from build123d import *

# Parameters (mm, degrees)
F0_W     = 1828.8
F0_H     = 558.8
F1_DEPTH = 19.05
F2_W     = 38.1
F2_H     = 88.9
F3_DEPTH = 1828.8
F4_W     = 38.1
F4_H     = 88.9
F5_DEPTH = 482.6
F6_W     = 88.9
F6_H     = 38.1
F7_DEPTH = 863.6


with BuildPart() as f1:
    # F0 (on Top) → F1 (new body)
    with BuildSketch(Plane.XY):
        with Locations((914.4, -279.4)):
            Rectangle(F0_W, F0_H)
    extrude(amount=F1_DEPTH)

    # F2 (on face) → F3 (join, through all)
    with BuildSketch(Plane.YZ.offset(1828.8)):
        with Locations((-539.75, -44.45)):
            Rectangle(F2_W, F2_H)
        with Locations((-19.05, -44.45)):
            Rectangle(F2_W, F2_H)
    extrude(amount=-F3_DEPTH)

    # F4 (on face) → F5 (join, through all)
    with BuildSketch(Plane.XZ.offset(38.1)):
        with Locations((19.05, -44.45)):
            Rectangle(F4_W, F4_H)
        with Locations((1809.75, -44.45)):
            Rectangle(F4_W, F4_H)
    extrude(amount=F5_DEPTH)

    # F6 (on face) → F7 (join)
    with BuildSketch(Plane(origin=(0, 0, 0), x_dir=(1, 0, 0), z_dir=(0, 0, -1))):
        with Locations((1746.25, 501.65)):
            Rectangle(F6_W, F6_H)
        with Locations((1746.25, 57.15)):
            Rectangle(F6_W, F6_H)
        with Locations((82.55, 57.15)):
            Rectangle(F6_W, F6_H)
        with Locations((82.55, 501.65)):
            Rectangle(F6_W, F6_H)
    extrude(amount=F7_DEPTH)


solid = f1.part
Verification items for the finished model (mm, model axes). A direction names the side the tool comes from. Give positions to 0.01 mm unless a question says otherwise; leave off trailing zeros. Loops run counter-clockwise (first coordinate to the right, second up) from the corner with the lowest first, then second, coordinate; pieces in that order, holes last.
1. Release check for a two-part mould opening along Y. For faces 1 (the flat face through (1746, -38.1, -471)), 2 (the flat face through (1790.7, -277, -45)), 3 (the flat face through (1746, -520.7, -471)) record: +Y half, -Y half, draft (parallel to the pull), parting line (faces both ways), or undercut.
Derived:
face 1: +Y half
face 2: undercut
face 3: -Y half
2. Tool access check on faces 4 (the flat face through (1746, -57, -863.6)), 5 (the flat face through (925, -38.1, -45)). Record the directions out of +Z, -Z, +X, -X, +Y, -Y that give a thin tool (end or side, any length) a straight path to the whole face; none if there is none.
Derived:
face 4: -Z, +X, -X, +Y, -Y
face 5: -Z
3. Cross-section at A-A on z = -780.5. Record the cut outline in (x, y).
Derived:
outline: (38.1, -520.7) - (127, -520.7) - (127, -482.6) - (38.1, -482.6) - close; (38.1, -76.2) - (127, -76.2) - (127, -38.1) - (38.1, -38.1) - close; (1701.8, -520.7) - (1790.7, -520.7) - (1790.7, -482.6) - (1701.8, -482.6) - close; (1701.8, -76.2) - (1790.7, -76.2) - (1790.7, -38.1) - (1701.8, -38.1) - close
4. Cross-section at C-C on y = -337. Record the cut outline in (x, z), and give its area (3 significant figures).
Derived:
outline: (0, -88.9) - (38.1, -88.9) - (38.1, 0) - (1790.7, 0) - (1790.7, -88.9) - (1828.8, -88.9) - (1828.8, 19.05) - (0, 19.05) - close
area: 41,600 mm2
5. Cross-section at B-B on x = 1049.5. Record the cut outline in (y, z).
Derived:
outline: (-558.8, -88.9) - (-520.7, -88.9) - (-520.7, 0) - (-38.1, 0) - (-38.1, -88.9) - (0, -88.9) - (0, 19.05) - (-558.8, 19.05) - close
6. Material ranges on probe 1 along X at (y, z) = (-57.5, -551); probe 2 along Z at (x, y) = (1525.5, -299); probe 3 along Y at (x, z) = (344.5, -24), recorded low to high.
Derived:
probe 1: x = 38.1 to 127, 1701.8 to 1790.7
probe 2: z = 0 to 19.05
probe 3: y = -558.8 to -520.7, -38.1 to 0
7. Go/stop test with flat-tipped pins: P1, Ø19, axis at y = -51, z = -478.5, coming from the +X side; P2, Ø1, axis at x = 1155.5, y = -267, coming from the -Z side; P3, Ø11.5, axis at y = -498.5, z = -323, coming from the -X side. Record where each tip stops, or that it passes through.
Derived:
P1: stops at x = 1790.7
P2: stops at z = 0
P3: stops at x = 38.1
